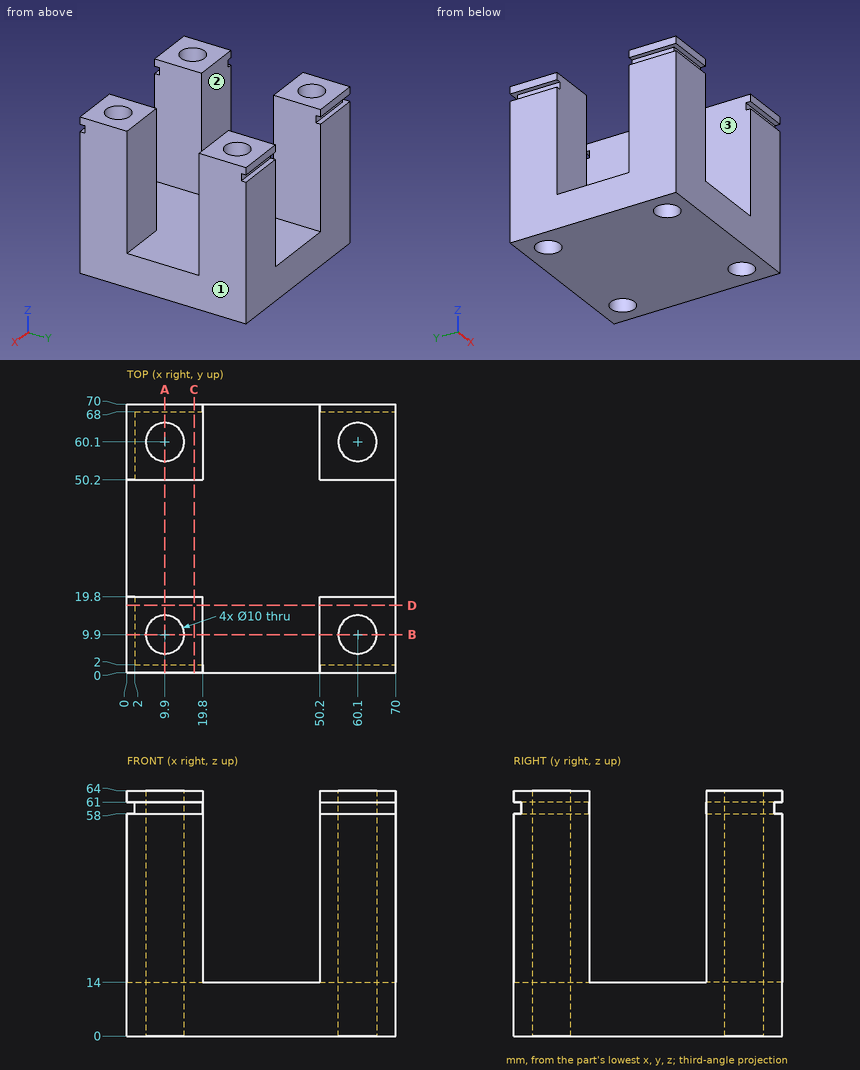
Could you check a few things on this drawing? It's one solid part, dimensions in mm from its lowest x, y, z. A direction names the side the tool comes from. Give positions to 0.01 mm unless a question says otherwise; leave off trailing zeros. Order: outer loops, then holes, each group sorted by start corner. A loop starts at its lowest first (then second) coordinate and runs counter-clockwise, first axis right, second up. Notation, with made-up numbers: (59, 31) - (69, 31) arc R10 cw to (69, 49) - close; hole circle Ø5 at (37, 46). An arc over 180 degrees is marked (long way). Return JSON: item names as keys, results as strings. Group by question number.
Q1. Please list where these lines run through material, in increasing order: line 1 along X through (y, z) = (60.1, 15.5); line 2 along Y through (x, z) = (63, 49.5); line 3 along X through (y, z) = (57, 46). Write a range as [from, to].
Q2. Which directions (+Z, -Z, +X, -X, +Y, -Y) give clear straight access to the entire face, cutting with the end or side of a thin tool? Please do the marked faces 1, 2 and 3.
Q3. Suppose I cut it at A-A, the plane x = 9.9. Please give me the cut outline in (y, z), and give its area (3 significant figures).
Q4. Will these pins go through, and if not, where does the flat tip stop? pin 1 Ø6 at (x, y) = (14.5, 6) entering from -Z; pin 2 Ø0.9 at (x, z) = (63, 59.5) entering from -Y; pin 3 Ø5 at (x, z) = (26, 17) entering from +Y; pin 4 Ø2.5 at (y, z) = (12, 59.5) entering from -X.
Q5. Suppose I cut it at D-D, the plane y = 17.5. Please give me the cut outline in (x, z), and give its area (3 significant figures).
Q6. Suppose I cut it at B-B, the plane y = 9.9. Please give me the cut outline in (x, z).
Q7. Suppose I cut it at C-C, the plane x = 17.5. Please give me the cut outline in (y, z).
Resolved:
{
 "1": {"line 1": "x = [0, 4.9], [14.9, 19.8], [50.2, 55.1], [65.1, 70]", "line 2": "y = [0, 5.83], [13.97, 19.8], [50.2, 56.03], [64.17, 70]", "line 3": "x = [0, 5.98], [13.82, 19.8], [50.2, 56.18], [64.02, 70]"},
 "2": {"face 1": "+Z, -Z, +X, +Y, -Y", "face 2": "+Z, +X, -X", "face 3": "+Z, +Y, -Y"},
 "3": {"outline": "(0, 0) - (4.9, 0) - (4.9, 64) - (0, 64) - (0, 61) - (2, 61) - (2, 58) - (0, 58) - close; (14.9, 0) - (55.1, 0) - (55.1, 64) - (50.2, 64) - (50.2, 14) - (19.8, 14) - (19.8, 64) - (14.9, 64) - close; (65.1, 0) - (70, 0) - (70, 58) - (68, 58) - (68, 61) - (70, 61) - (70, 64) - (65.1, 64) - close", "area": "1,670 mm2"},
 "4": {"pin 1": "stops at z = 0", "pin 2": "stops at y = 2", "pin 3": "passes through", "pin 4": "stops at x = 2"},
 "5": {"outline": "(0, 0) - (70, 0) - (70, 64) - (50.2, 64) - (50.2, 14) - (19.8, 14) - (19.8, 64) - (0, 64) - (0, 61) - (2, 61) - (2, 58) - (0, 58) - close", "area": "2,950 mm2"},
 "6": {"outline": "(0, 0) - (4.9, 0) - (4.9, 64) - (0, 64) - (0, 61) - (2, 61) - (2, 58) - (0, 58) - close; (14.9, 0) - (55.1, 0) - (55.1, 64) - (50.2, 64) - (50.2, 14) - (19.8, 14) - (19.8, 64) - (14.9, 64) - close; (65.1, 0) - (70, 0) - (70, 64) - (65.1, 64) - close"},
 "7": {"outline": "(0, 0) - (70, 0) - (70, 58) - (68, 58) - (68, 61) - (70, 61) - (70, 64) - (50.2, 64) - (50.2, 14) - (19.8, 14) - (19.8, 64) - (0, 64) - (0, 61) - (2, 61) - (2, 58) - (0, 58) - close"}
}
